```python
from build123d import *

# Parameters (mm, degrees)
EXTRUDE_1_DEPTH = 4


with BuildPart() as part:
    # 草图1 → 凸台-拉伸1 (new body)
    with BuildSketch(Plane.XY):
        Polygon((0, 0), (0, -4), (-1.35, -4), (-1.35, -6.6), (0, -6.6), (0, -8.6), (3, -8.6), (3, -6.6), (4.35, -6.6), (4.35, -4), (3, -4), (3, 0), (30.5, 0), (30.5, 4), (38.5, 4), (38.5, 0), (66, 0), (66, -4), (64.65, -4), (64.65, -6.6), (66, -6.6), (66, -8.6), (69, -8.6), (69, -6.6), (70.35, -6.6), (70.35, -4), (69, -4), (69, 0), (96.5, 0), (96.5, 4), (104.5, 4), (104.5, 0), (132, 0), (143.5, 0), (143.5, -63), (147.5, -63), (147.5, -71), (143.5, -71), (143.5, -98.5), (139.5, -98.5), (139.5, -97.15), (136.9, -97.15), (136.9, -98.5), (134.9, -98.5), (134.9, -101.5), (136.9, -101.5), (136.9, -102.85), (139.5, -102.85), (139.5, -101.5), (143.5, -101.5), (143.5, -129), (147.5, -129), (147.5, -137), (143.5, -137), (143.5, -200), (132, -200), (104.5, -200), (104.5, -204), (96.5, -204), (96.5, -200), (69, -200), (69, -196), (70.35, -196), (70.35, -193.4), (69, -193.4), (69, -191.4), (66, -191.4), (66, -193.4), (64.65, -193.4), (64.65, -196), (66, -196), (66, -200), (38.5, -200), (38.5, -204), (30.5, -204), (30.5, -200), (3, -200), (3, -196), (4.35, -196), (4.35, -193.4), (3, -193.4), (3, -191.4), (0, -191.4), (0, -193.4), (-1.35, -193.4), (-1.35, -196), (0, -196), (0, -200), (-27.5, -200), (-27.5, -204), (-35.5, -204), (-35.5, -200), (-63, -200), (-63, -196), (-61.65, -196), (-61.65, -193.4), (-63, -193.4), (-63, -191.4), (-66, -191.4), (-66, -193.4), (-67.35, -193.4), (-67.35, -196), (-66, -196), (-66, -200), (-93.5, -200), (-93.5, -204), (-101.5, -204), (-101.5, -200), (-129, -200), (-140.5, -200), (-140.5, -137), (-144.5, -137), (-144.5, -129), (-140.5, -129), (-140.5, -101.5), (-136.5, -101.5), (-136.5, -102.85), (-133.9, -102.85), (-133.9, -101.5), (-131.9, -101.5), (-131.9, -98.5), (-133.9, -98.5), (-133.9, -97.15), (-136.5, -97.15), (-136.5, -98.5), (-140.5, -98.5), (-140.5, -71), (-144.5, -71), (-144.5, -63), (-140.5, -63), (-140.5, 0), (-129, 0), (-101.5, 0), (-101.5, 4), (-93.5, 4), (-93.5, 0), (-66, 0), (-66, -4), (-67.35, -4), (-67.35, -6.6), (-66, -6.6), (-66, -8.6), (-63, -8.6), (-63, -6.6), (-61.65, -6.6), (-61.65, -4), (-63, -4), (-63, 0), (-35.5, 0), (-35.5, 4), (-27.5, 4), (-27.5, 0), align=None)
    extrude(amount=EXTRUDE_1_DEPTH)


solid = part.part
```
The model under review builds one solid part; all positions refer to its coordinate system, in mm. Coordinates: 2 decimals unless noted, no trailing zeros. Write each loop counter-clockwise with the first axis right and the second up, starting at its lowest first coordinate (ties: lowest second). Pieces come first, ordered by that corner, then holes. Notation, with made-up numbers: (43, -23) - (79, -23) arc R18 cw to (79, -7) - close; hole circle Ø1 at (19.25, 75). An arc over 180 degrees is marked (long way). Answer in a Markdown table with one row per item. Add a question column.
Q1. Clearance check with flat-ended pins moving along their axes: pin 1 (1.5 mm diameter, centred on y = -98, z = 1, fed in from -X); pin 2 (0.6 mm diameter, centred on y = -193, z = 3, fed in from +X); pin 3 (3 mm diameter, centred on x = 101.5, y = -69.5, fed in from -Z); pin 4 (2 mm diameter, centred on x = 115.5, z = 1.5, fed in from -Y). State where each tip first meets the part, or that it passes through.
Q2. Consider section A-A on y = -57. Give the boundary of the cut face in (x, z), then the cut area to 3 significant figures.
Q3. Consider section B-B on x = 75. Give the boundary of the cut face in (y, z).
Q4. To check wall thickness, follow line 1 along Y through (x, z) = (-109.5, 2); line 2 along X through (y, z) = (-30, 2.9). State the ranges of each line that lie inside material, in increasing order. Write a range as from..to.
Answers below:
| question | item | result |
|---|---|---|
| 1 | pin 1 | x = -140.5 |
| 1 | pin 2 | x = 143.5 |
| 1 | pin 3 | z = 0 |
| 1 | pin 4 | y = -200 |
| 2 | outline | (-140.5, 0) - (143.5, 0) - (143.5, 4) - (-140.5, 4) - close |
| 2 | area | 1,140 mm² |
| 3 | outline | (-200, 0) - (0, 0) - (0, 4) - (-200, 4) - close |
| 4 | line 1 | -200..0 |
| 4 | line 2 | -140.5..143.5 |
